Verification items for the finished model (mm, model axes). A direction names the side the tool comes from. Give positions to 0.01 mm unless a question says otherwise; leave off trailing zeros. Loops run counter-clockwise (first coordinate to the right, second up) from the corner with the lowest first, then second, coordinate; pieces in that order, holes last. Notation, with made-up numbers: M 48.5,54 L 107.5,54 A30 ccw 107.5,83 Z; hole C 20.25,83 d5. An arc over 180 degrees is marked long. Answer in a Markdown table with one row per item.
```python
from build123d import *

# Parameters (mm, degrees)
F0_W     = 480
F0_H     = 200
F1_DEPTH = 8


with BuildPart() as f1:
    # F0 (on Right) → F1 (new body)
    with BuildSketch(Plane.YZ):
        with Locations((-37.386954, 100)):
            Rectangle(F0_W, F0_H)
        Polygon((-247.386954, 30), (-247.386954, 170), (-107.386954, 170), (32.613046, 170), (172.613046, 170), (172.613046, 30), (32.613046, 30), (-107.386954, 30), align=None, mode=Mode.SUBTRACT)
    extrude(amount=F1_DEPTH)


solid = f1.part
```
Item 1: Sectioned sample at C-C (x = 2.25). Record the cut outline in (y, z).
Reported:
| item | result |
|---|---|
| outline | M -277.39,0 L 202.61,0 L 202.61,200 L -277.39,200 Z; hole M -247.39,30 L 172.61,30 L 172.61,170 L -247.39,170 Z |
Item 2: Sectioned sample at B-B (z = 72). Record the cut outline in (x, y).
Reported:
| item | result |
|---|---|
| outline | M 0,-277.39 L 8,-277.39 L 8,-247.39 L 0,-247.39 Z; M 0,172.61 L 8,172.61 L 8,202.61 L 0,202.61 Z |
Item 3: Tool access check on faces 1 (the flat face through (4, 202.613, 99)), 2 (the flat face through (4, -40, 170)). Record the directions out of +Z, -Z, +X, -X, +Y, -Y that give a thin tool (end or side, any length) a straight path to the whole face; none if there is none.
Reported:
| item | result |
|---|---|
| face 1 | +Z, -Z, +X, -X, +Y |
| face 2 | +X, -X |
Item 4: Release check for a two-part mould opening along Z. For faces 3 (the flat face through (0, -56, 26)), 4 (the flat face through (4, -34, 30)), 5 (the flat face through (4, -41, 200)) record: released by +Z, released by -Z, zero draft, split by the parting line, or undercut.
Reported:
| item | result |
|---|---|
| face 3 | zero draft |
| face 4 | undercut |
| face 5 | released by +Z |
Item 5: Sectioned sample at A-A (y = -104). Record the cut outline in (x, z).
Reported:
| item | result |
|---|---|
| outline | M 0,0 L 8,0 L 8,30 L 0,30 Z; M 0,170 L 8,170 L 8,200 L 0,200 Z |
Item 6: Scan lines: L1, parallel to Z at x = 1.5, y = -174; L2, parallel to Y at x = 4.75, z = 152.5. Record each from-to range of solid material in increasing order. Write a range as [from, to].
Reported:
| item | result |
|---|---|
| L1 | z = [0, 30], [170, 200] |
| L2 | y = [-277.39, -247.39], [172.61, 202.61] |
Item 7: Go/stop test with a flat-tipped pin: pin 1 (1 mm diameter, centred on x = 6, y = 30.5, fed in from -Z). Record where the tip stops, or that it passes through.
Reported:
| item | result |
|---|---|
| pin 1 | stops at z = 0 |
